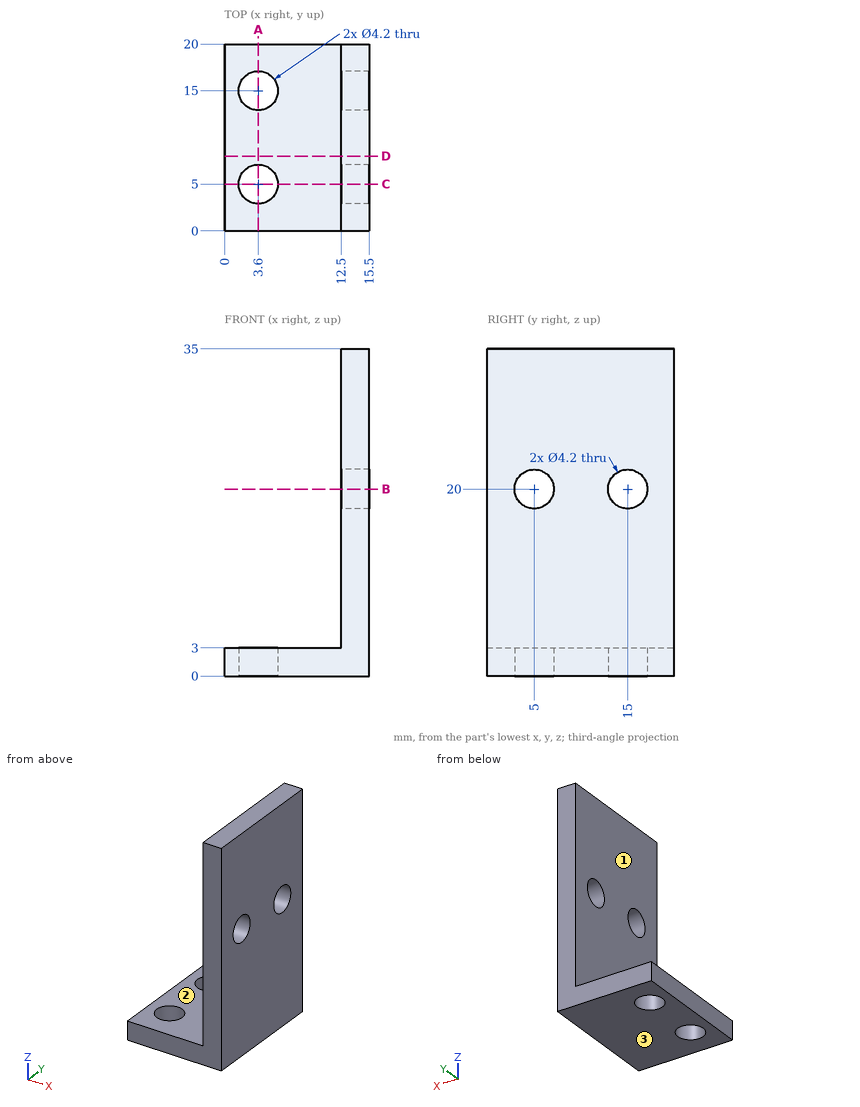
Job drawing, mm, ordinate dimensions from the low corner. One solid piece. Coordinates: 2 decimals unless noted, no trailing zeros. Order: outer loops, then holes, each group sorted by start corner. A loop starts at its lowest first (then second) coordinate and runs counter-clockwise, first axis right, second up. Notation, with made-up numbers: (10, -16) - (65, -16) arc R36 cw to (65, 18) - close; hole circle Ø2 at (49, 88.25). An arc over 180 degrees is marked (long way). Use CSV: the item, a comma, the result in double quotes.
Item 1: Saw through at B-B on z = 20. Give the cut face in (x, y), and give its area (3 significant figures).
Solved:
outline,"(12.5, 0) - (15.5, 0) - (15.5, 2.9) - (12.5, 2.9) - close; (12.5, 7.1) - (15.5, 7.1) - (15.5, 12.9) - (12.5, 12.9) - close; (12.5, 17.1) - (15.5, 17.1) - (15.5, 20) - (12.5, 20) - close"
area,"34.8 mm²"
Item 2: Saw through at D-D on y = 8. Give the cut face in (x, z), and give its area (4 significant figures).
Solved:
outline,"(0, 0) - (15.5, 0) - (15.5, 35) - (12.5, 35) - (12.5, 3) - (0, 3) - close"
area,"142.5 mm²"
Item 3: Saw through at A-A on x = 3.6. Give the cut face in (y, z).
Solved:
outline,"(0, 0) - (2.9, 0) - (2.9, 3) - (0, 3) - close; (7.1, 0) - (12.9, 0) - (12.9, 3) - (7.1, 3) - close; (17.1, 0) - (20, 0) - (20, 3) - (17.1, 3) - close"
Item 4: Drop flat-ended pins along their axis: P1, Ø1.5, axis at x = 10, y = 14, coming from the +Z side; P2, Ø5.5, axis at y = 15, z = 20, coming from the -X side; P3, Ø2, axis at x = 4.5, y = 6.5, coming from the -Z side; P4, Ø4, axis at y = 5, z = 20, coming from the -X side. Give the stop position or say it passes through.
Solved:
P1,"stops at z = 3"
P2,"stops at x = 12.5"
P3,"stops at z = 0"
P4,"passes through"
Item 5: Mould opens along Z. For the marked faces 1, 2 and 3 say: +Z half, -Z half, draft (parallel to the pull), parting line (faces both ways), or undercut.
Solved:
face 1,"draft"
face 2,"+Z half"
face 3,"-Z half"
Item 6: Probe probe 1 along Y at (x, z) = (3.6, 0.95); probe 2 along X at (y, z) = (15.5, 5.5); probe 3 along Z at (x, y) = (6.5, 4.75). List the from-to ranges inside material, lowest first.
Solved:
probe 1,"y = 0 to 2.9, 7.1 to 12.9, 17.1 to 20"
probe 2,"x = 12.5 to 15.5"
probe 3,"z = 0 to 3"
Item 7: Saw through at C-C on y = 5. Give the cut face in (x, z).
Solved:
outline,"(0, 0) - (1.5, 0) - (1.5, 3) - (0, 3) - close; (5.7, 0) - (15.5, 0) - (15.5, 17.9) - (12.5, 17.9) - (12.5, 3) - (5.7, 3) - close; (12.5, 22.1) - (15.5, 22.1) - (15.5, 35) - (12.5, 35) - close"
